Autodesk Inventor part; units mm, degrees
ref_plane "Work Plane1" through (0, 41.5, 0) normal (0, 1, 0) x (1, 0, 0)
ref_plane "Work Plane2" through (0, 50.2, 0) normal (0, 1, 0) x (1, 0, 0)
ref_plane "YZ Plane" through (0, 0, 0) normal (1, 0, 0) x (0, 1, 0)
sketch "Sketch1" plane through (0, 0, 0) normal (0, 1, 0) x (-1, 0, 0)
  circle A0 centre (0, 0) radius 13.7
  dimension "d0" = 27.4
extrude "Extrusion1" add sketch "Sketch1" along normal blind 46.5
sketch "Sketch2" plane through (0, 46.5, 0) normal (0, 1, 0) x (1, 0, 0)
  circle A0 centre (0, 0) radius 13.7
  circle A1 centre (0, 0) radius 5
  dimension "d3" = 10
extrude "Extrusion2" add sketch "Sketch2" along normal blind 2.7 contours A1
sketch "Sketch3" plane through (0, 46.5, 0) normal (0, 1, 0) x (1, 0, 0)
  circle A0 centre (0, 0) radius 5
  circle A1 centre (0, 0) radius 5
  circle A2 centre (0, 0) radius 13.7
  circle A3 centre (0, 0) radius 13.7
  line L0 (-13.7, 0) -> (13.7, 0)
  point P0 (-8, 0)
  point P1 (8, 0)
  dimension "d6" = 16
  dimension "d7" = 5.7
  dimension "d8" = 5.7
hole "Hole1" at (-8, 46.5, 0) at (8, 46.5, 0) direction (0, -1, 0) diameter 2.1129 depth 2.8
ref_plane "Work Plane1" through (0, 41.5, 0) normal (0, 1, 0) x (1, 0, 0)
sketch "Sketch4" plane through (0, 41.5, 0) normal (0, 1, 0) x (1, 0, 0)
  circle A0 centre (0, 0) radius 14.375
  dimension "d17" = 28.75
extrude "Extrusion3" add sketch "Sketch4" against normal blind 27.7
sketch "Sketch5" plane through (0, 0, 0) normal (0, -1, 0) x (1, 0, 0)
  circle A0 centre (0, 0) radius 5
  dimension "d20" = 10
extrude "Extrusion4" add sketch "Sketch5" along normal blind 4
sketch "Sketch6" plane through (0, 0, 0) normal (0, -1, 0) x (1, 0, 0)
  circle A0 centre (0, 0) radius 5
  circle A1 centre (0, 0) radius 5
  circle A2 centre (0, 0) radius 13.7
  circle A3 centre (0, 0) radius 13.7
  line L0 (13.7, 0) -> (-13.7, 0)
  line L1 (-11.5, 1.5) -> (-12, 1.5)
  line L2 (-12, 1.5) -> (-12, -1.5)
  line L3 (-12, -1.5) -> (-11.5, -1.5)
  line L4 (-11.5, -1.5) -> (-11.5, 1.5)
  line L5 (11.5, 1.5) -> (11, 1.5)
  line L6 (11, 1.5) -> (11, -1.5)
  line L7 (11, -1.5) -> (11.5, -1.5)
  line L8 (11.5, -1.5) -> (11.5, 1.5)
  dimension "d23" = 22.5
  dimension "d24" = 0.5
  dimension "d25" = 0.5
  dimension "d26" = 11.5
  dimension "d27" = 11.5
  dimension "d28" = 3
  dimension "d29" = 3
  dimension "d30" = 1.5
  dimension "d31" = 1.5
extrude "Extrusion5" add sketch "Sketch6" along normal blind 6 contours L6 L5 L8 L0 | L0 L8 L7 L6 | L4 L3 L2 L0 | L0 L2 L1 L4
sketch "Sketch7" plane through (0, 49.2, 0) normal (0, 1, 0) x (1, 0, 0)
  circle A0 centre (0, 0) radius 1.1
  dimension "d34" = 2.2
extrude "Extrusion6" add sketch "Sketch7" along normal blind 13.5
ref_plane "Work Plane2" through (0, 50.2, 0) normal (0, 1, 0) x (1, 0, 0)
equation "\"d26\" = d27"
equation "\"d30\" = d31"
equation "\"d41\" = d42"
properties part number "rs390" material "Steel, Mild"
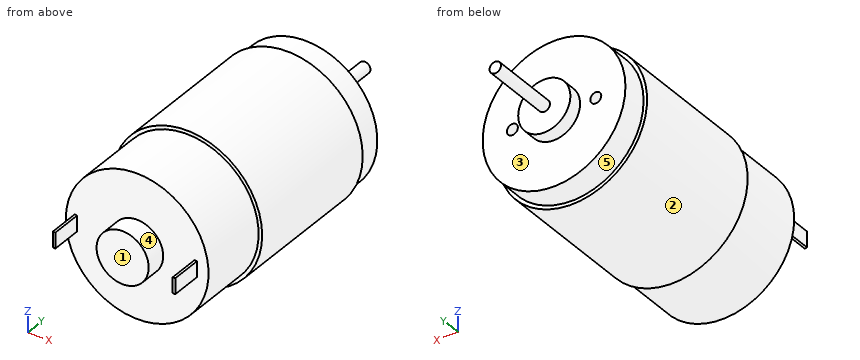
Source: CAD feature listing. Evaluate the final solid. Frame: model axes, mm. Face numbers are marked on the shaded views. A direction names the side the tool comes from. Round coordinates to 2 decimals unless told otherwise and drop trailing zeros. Loops run counter-clockwise (first coordinate to the right, second up) from the corner with the lowest first, then second, coordinate; pieces in that order, holes last. Notation, with made-up numbers: M 10.25,35 L 69.25,35 A13 cw 69.25,56 Z; hole C 49,44.5 d10. An arc over 180 degrees is marked long. Use a Markdown table: item, result. Add a question column.
1. Mould query, pull axis X, two halves, no side actions, for the marked faces 1, 2 and 3. Classes: pulls with the +X half, pulls with the -X half, needs draft (parallel to the pull), parting line crosses it, or undercut.
2. Reachability of the marked faces 4 and 5 from +Z, -Z, +X, -X, +Y, -Y: full face, straight path, thin tool, end or side. Return the list, or none.
3. Contact query for flat-ended pins moving along their axis: P1, Ø1.7, axis at x = -8, z = 0, coming from the -Y side; P2, Ø10, axis at y = 9.5, z = 8, coming from the -X side; P3, Ø3, axis at y = 17.5, z = -4, coming from the -X side; P4, Ø3, axis at x = 1.5, z = 0.5, coming from the +Y side. Output: stop coordinate, or through.
4. Section query C-C on y = 56.5. Return the cut outline in (x, z).
5. Section query A-A on x = 0. Return the cut outline in (y, z) (3 decimals), then the cut area to 3 significant figures.
6. Line query: line 1 (X direction, y = 45, z = 0); line 2 (Y direction, x = -0.25, z = 9.5); line 3 (Y direction, x = -10.5, z = 9). Output: solid intervals per line, ascending.
7. Section query D-D on x = 3. Return the cut outline in (y, z), then the cut area to 3 significant figures.
8. Section query B-B on z = 2.25. Return the cut outline in (x, y), then the cut area to 3 significant figures.
Reported:
| question | item | result |
|---|---|---|
| 1 | face 1 | undercut |
| 1 | face 2 | parting line crosses it |
| 1 | face 3 | needs draft |
| 2 | face 4 | -Y |
| 2 | face 5 | +Y |
| 3 | P1 | stops at y = 0 |
| 3 | P2 | stops at x = -13.37 |
| 3 | P3 | stops at x = -14.16 |
| 3 | P4 | stops at y = 62.7 |
| 4 | outline | C 0,0 d2.2 |
| 5 | outline | M -4,-5 L 0,-5 L 0,-13.7 L 13.8,-13.7 L 13.8,-14.375 L 41.5,-14.375 L 41.5,-13.7 L 46.5,-13.7 L 46.5,-5 L 49.2,-5 L 49.2,-1.1 L 62.7,-1.1 L 62.7,1.1 L 49.2,1.1 L 49.2,5 L 46.5,5 L 46.5,13.7 L 41.5,13.7 L 41.5,14.375 L 13.8,14.375 L 13.8,13.7 L 0,13.7 L 0,5 L -4,5 Z |
| 5 | area | 1,410 mm² |
| 6 | line 1 | x = -13.7 to -9.06, -6.94 to 6.94, 9.06 to 13.7 |
| 6 | line 2 | y = 0 to 46.5 |
| 6 | line 3 | y = 13.8 to 41.5 |
| 7 | outline | M -4,-4 L 0,-4 L 0,-13.37 L 13.8,-13.37 L 13.8,-14.06 L 41.5,-14.06 L 41.5,-13.37 L 46.5,-13.37 L 46.5,-4 L 49.2,-4 L 49.2,4 L 46.5,4 L 46.5,13.37 L 41.5,13.37 L 41.5,14.06 L 13.8,14.06 L 13.8,13.37 L 0,13.37 L 0,4 L -4,4 Z |
| 7 | area | 1,340 mm² |
| 8 | outline | M -14.2,13.8 L -13.51,13.8 L -13.51,0 L -4.47,0 L -4.47,-4 L 4.47,-4 L 4.47,0 L 13.51,0 L 13.51,13.8 L 14.2,13.8 L 14.2,41.5 L 13.51,41.5 L 13.51,46.5 L 4.47,46.5 L 4.47,49.2 L -4.47,49.2 L -4.47,46.5 L -13.51,46.5 L -13.51,41.5 L -14.2,41.5 Z |
| 8 | area | 1,350 mm² |
